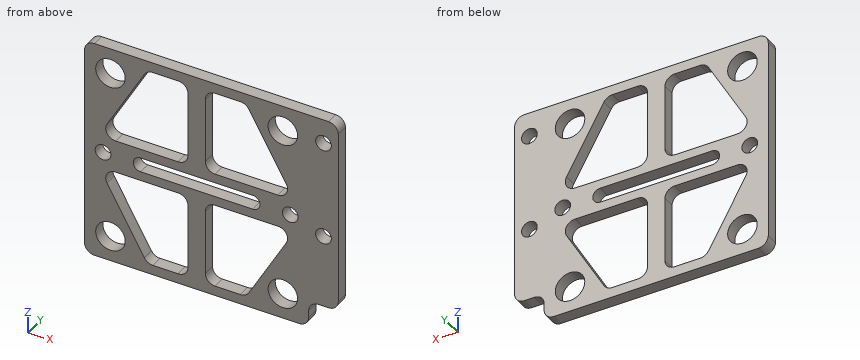
from build123d import *

# Parameters (mm, degrees)
SKETCH_1_W          = 45.5
SKETCH_1_H          = 45.5
SKETCH_1_R          = 3
EXTRUDE_1_DEPTH     = 2.5
SKETCH_2_W          = 6
SKETCH_2_H          = 40
SKETCH_2_R          = 1.6
EXTRUDE_2_DEPTH     = 2.5
FILLET_1_R          = 2
CUT_EXTRUDE_1_DEPTH = 37.747448891
FILLET_2_R          = 2
SKETCH_4_R          = 1.6
CUT_EXTRUDE_2_DEPTH = 37.747448891


with BuildPart() as part:
    # 草图1 → 凸台-拉伸1 (new body)
    with BuildSketch(Plane(origin=(0, 0, 0), x_dir=(1, 0, 0), z_dir=(0, 1, 0))):
        Rectangle(SKETCH_1_W, SKETCH_1_H)
        with Locations(Location((17.5, 17.5, 0), (0, 0, 270))):
            Circle(SKETCH_1_R, mode=Mode.SUBTRACT)
        with Locations(Location((17.5, -17.5, 0), (0, 0, 270))):
            Circle(SKETCH_1_R, mode=Mode.SUBTRACT)
        with Locations(Location((-17.5, -17.5, 0), (0, 0, 90))):
            Circle(SKETCH_1_R, mode=Mode.SUBTRACT)
        with Locations(Location((-17.5, 17.5, 0), (0, 0, 90))):
            Circle(SKETCH_1_R, mode=Mode.SUBTRACT)
    extrude(amount=EXTRUDE_1_DEPTH)

    # 草图2 → 凸台-拉伸2 (add)
    with BuildSketch(Plane(origin=(0, 2.5, 0), x_dir=(1, 0, 0), z_dir=(0, 1, 0))):
        with Locations((25.75, -2.75)):
            Rectangle(SKETCH_2_W, SKETCH_2_H)
        with Locations(Location((25.75, -17.75, 0), (0, 0, 270))):
            Circle(SKETCH_2_R, mode=Mode.SUBTRACT)
        with Locations(Location((25.75, 2.25, 0), (0, 0, 270))):
            Circle(SKETCH_2_R, mode=Mode.SUBTRACT)
    extrude(amount=-EXTRUDE_2_DEPTH)

    # 圆角1
    fillet_1_edges = [part.edges().sort_by_distance(p)[0] for p in [
        (28.75, 1.25, -17.25),
        (22.75, 1.25, -17.25),
        (28.75, 1.25, 22.75),
        (-22.75, 1.25, 22.75),
        (-22.75, 1.25, -22.75),
        (22.75, 1.25, -22.75),
    ]]
    fillet(fillet_1_edges, radius=FILLET_1_R)

    # 草图3 → 切除-拉伸1 (cut, through all)
    with BuildSketch(Plane(origin=(0, 2.5, 0), x_dir=(1, 0, 0), z_dir=(0, 1, 0))):
        Polygon((-10.045962714, 20.729282101), (-19.893887011, 3.33704153), (-1.766794069, 3.33704153), (-1.766794069, 20.729282101), align=None)
        Polygon((1.766794069, 3.33704153), (1.766794069, 20.729282101), (10.045962714, 20.729282101), (19.893887011, 3.33704153), align=None)
        Polygon((19.893887011, -3.33704153), (1.766794069, -3.33704153), (1.766794069, -20.729282101), (10.045962714, -20.729282101), align=None)
        Polygon((-1.766794069, -3.33704153), (-1.766794069, -20.729282101), (-10.045962714, -20.729282101), (-19.893887011, -3.33704153), align=None)
        with BuildLine():
            Line((-11.375, 1.5), (11.375, 1.5))
            ThreePointArc((11.375, 1.5), (12.875, 0), (11.375, -1.5))
            Line((11.375, -1.5), (-11.375, -1.5))
            ThreePointArc((-11.375, -1.5), (-12.875, 0), (-11.375, 1.5))
        make_face()
    extrude(amount=-CUT_EXTRUDE_1_DEPTH, mode=Mode.SUBTRACT)

    # 圆角2
    fillet_2_edges = [part.edges().sort_by_distance(p)[0] for p in [
        (19.893887011, 1.25, -3.33704153),
        (1.766794069, 1.25, -3.33704153),
        (1.766794069, 1.25, -20.729282101),
        (10.045962714, 1.25, -20.729282101),
        (19.893887011, 1.25, 3.33704153),
        (10.045962714, 1.25, 20.729282101),
        (1.766794069, 1.25, 20.729282101),
        (1.766794069, 1.25, 3.33704153),
        (-19.893887011, 1.25, 3.33704153),
        (-1.766794069, 1.25, 3.33704153),
        (-1.766794069, 1.25, 20.729282101),
        (-10.045962714, 1.25, 20.729282101),
        (-10.045962714, 1.25, -20.729282101),
        (-1.766794069, 1.25, -20.729282101),
        (-1.766794069, 1.25, -3.33704153),
        (-19.893887011, 1.25, -3.33704153),
    ]]
    fillet(fillet_2_edges, radius=FILLET_2_R)

    # 草图4 → 切除-拉伸2 (cut, through all)
    with BuildSketch(Plane(origin=(0, 2.5, 0), x_dir=(1, 0, 0), z_dir=(0, 1, 0))):
        with Locations(Location((-19, 0, 0), (0, 0, 270))):
            Circle(SKETCH_4_R)
        with Locations(Location((19, 0, 0), (0, 0, 90))):
            Circle(SKETCH_4_R)
    extrude(amount=-CUT_EXTRUDE_2_DEPTH, mode=Mode.SUBTRACT)


solid = part.part
Design review of the part built by this model. Coordinates are the model's own, in mm. Give positions to 0.01 mm unless a question says otherwise; leave off trailing zeros. Loops run counter-clockwise (first coordinate to the right, second up) from the corner with the lowest first, then second, coordinate; pieces in that order, holes last. Notation, with made-up numbers: M -10.5,66.25 L 11.5,66.25 A33 ccw 11.5,101.25 Z; hole C 37,5.25 d1. An arc over 180 degrees is marked long. Write item = value, one per line.
Q1. We need section C-C (z = 17.75). Give the boundary of the cut face in (x, y), plus the area to 3 significant figures.
Output values:
outline = M -22.75,0 L -20.49,0 L -20.49,2.5 L -22.75,2.5 Z; M -14.51,0 L -11.73,0 L -11.73,2.5 L -14.51,2.5 Z; M -1.77,0 L 1.77,0 L 1.77,2.5 L -1.77,2.5 Z; M 11.73,0 L 14.51,0 L 14.51,2.5 L 11.73,2.5 Z; M 20.49,0 L 24.15,0 L 24.15,2.5 L 20.49,2.5 Z; M 27.35,0 L 28.75,0 L 28.75,2.5 L 27.35,2.5 Z
area = 41.0 mm^2
Q2. To check wall thickness, follow line 1 (Z direction, x = -4, y = 2.05); line 2 (X direction, y = 0.75, z = -5.5); line 3 (Z direction, x = 2, y = 1.9). State the ranges of each line that lie inside material, in increasing order. Write a range as [from, to].
Output values:
line_1 = [-22.75, -20.73], [-3.34, -1.5], [1.5, 3.34], [20.73, 22.75]
line_2 = [-22.75, -18.46], [-1.77, 1.77], [18.46, 28.75]
line_3 = [-22.75, -19.67], [-4.4, -1.5], [1.5, 4.4], [19.67, 22.75]
Q3. We need section D-D (y = 1.4). Count the separate pieces of the cut face and the enclosed holes in it, plus the area to 3 significant figures.
Output values:
separate_pieces = 1
enclosed_holes = 13
area = 1,190 mm^2
Q4. We need section B-B (x = 25.75). Give the boundary of the cut face in (y, z), plus the area to 3 significant figures.
Output values:
outline = M 0,-17.25 L 2.5,-17.25 L 2.5,-3.85 L 0,-3.85 Z; M 0,-0.65 L 2.5,-0.65 L 2.5,16.15 L 0,16.15 Z; M 0,19.35 L 2.5,19.35 L 2.5,22.75 L 0,22.75 Z
area = 84.0 mm^2
Q5. Insertion check: pin 1 (1 mm diameter, centred on x = 25.5, y = 1, fed in from -Z). The pin has a flat end and moves straight along its axis. Give the tip position at first contact, or say it passes through.
Output values:
pin_1 = -17.25
Q6. We need section A-A (z = 0). Give the boundary of the cut face in (x, y) (3 decimals), plus the area to 3 significant figures.
Output values:
outline = M -22.75,0 L -20.6,0 L -20.6,2.5 L -22.75,2.5 Z; M -17.4,0 L -12.875,0 L -12.875,2.5 L -17.4,2.5 Z; M 12.875,0 L 17.4,0 L 17.4,2.5 L 12.875,2.5 Z; M 20.6,0 L 28.75,0 L 28.75,2.5 L 20.6,2.5 Z
area = 48.4 mm^2
